```python
from build123d import *


with BuildPart() as part:
    # Sketch2 → Revolve1 (revolve)
    with BuildSketch(Plane.XY, mode=Mode.PRIVATE) as revolve1_sk:
        with BuildLine():
            Line((0, 0), (0, 2.175))
            ThreePointArc((0, 2.175), (-0.292893219, 2.882106781), (-1, 3.175))
            Line((-1, 3.175), (-1.3716, 3.175))
            Line((-1.3716, 3.175), (-1.3716, 1.63195))
            Line((-1.3716, 1.63195), (-7.7216, 1.63195))
            Line((-7.7216, 1.63195), (-7.7216, 2.43195))
            ThreePointArc((-7.7216, 2.43195), (-7.838757288, 2.714792712), (-8.1216, 2.83195))
            Line((-8.1216, 2.83195), (-8.3216, 2.83195))
            ThreePointArc((-8.3216, 2.83195), (-8.604442712, 2.714792712), (-8.7216, 2.43195))
            Line((-8.7216, 2.43195), (-8.7216, 2.38195))
            ThreePointArc((-8.7216, 2.38195), (-8.941269914, 1.851619914), (-9.4716, 1.63195))
            Line((-9.4716, 1.63195), (-9.764947502, 1.63195))
            ThreePointArc((-9.764947502, 1.63195), (-9.895473695, 1.623394861), (-10.023766548, 1.597875826))
            Line((-10.023766548, 1.597875826), (-10.526009523, 1.463300227))
            ThreePointArc((-10.526009523, 1.463300227), (-10.79327667, 1.284718028), (-10.8966, 0.980337314))
            Line((-10.8966, 0.980337314), (-10.8966, 0))
            Line((-10.8966, 0), (0, 0))
        make_face()
    revolve(revolve1_sk.sketch.rotate(Axis((-42.300017882, 0, 0), (1, 0, 0)), 90), axis=Axis((-42.300017882, 0, 0), (1, 0, 0)))


solid = part.part
```
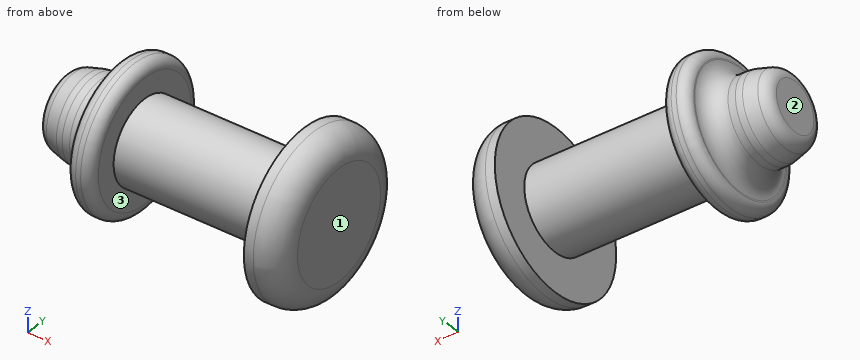
Here's how the part is built. I have some questions about the finished solid (model axes, mm). Face numbers are marked on the shaded views. Coordinates: 2 decimals unless noted, no trailing zeros. Write each loop counter-clockwise with the first axis right and the second up, starting at its lowest first coordinate (ties: lowest second). Pieces come first, ordered by that corner, then holes. Notation, with made-up numbers: M 89.5,-26.5 L 101.5,-26.5 A21 ccw 101.5,-13.5 Z; hole C -38,53.25 d11. An arc over 180 degrees is marked long. Answer as CSV lines item,"result". Start each with the question number.
Q1. Suppose I cut it at B-B, the plane x = -0.5. List the corners of the cut face in (y, z) for me.
Q2. I need wall thicknesses on probe 1 along X at (y, z) = (-1.5, -1.25); probe 2 along X at (y, z) = (-1, -0.25); probe 3 along X at (y, z) = (2, 1.5). Which ranges of each line are inside material? Lowest first, please. Write a range as [from, to].
Q3. Will these pins go through, and if not, where does the flat tip stop? pin 1 Ø1.5 at (x, z) = (-1.5, -1) entering from -Y; pin 2 Ø2 at (x, z) = (-5, -1) entering from +Y; pin 3 Ø2 at (x, y) = (-2.5, 2) entering from +Z; pin 4 Ø1.5 at (x, z) = (-4.5, -2.5) entering from -Y.
Q4. Suppose I cut it at A-A, the plane x = -7.25. List the corners of the cut face in (y, z) for me, then the cut area to 3 significant figures.
Q5. If we mould it in two halves opening along X, with no side actions, what happens to the marked faces 1, 2 and 3? For each: pulls with the +X half, pulls with the -X half, needs draft (parallel to the pull), parting line crosses it, or undercut.
Entries:
1,outline,"C 0,0 d6.08"
2,probe 1,"x = [-8.86, -7.72], [-1.37, 0]"
2,probe 2,"x = [-10.89, 0]"
2,probe 3,"x = [-8.72, -7.73], [-1.37, -0.05]"
3,pin 1,"stops at y = -3.16"
3,pin 2,"stops at y = 1.63"
3,pin 3,"stops at z = 1.29"
3,pin 4,"passes through"
4,outline,"C 0,0 d3.26"
4,area,"8.37 mm²"
5,face 1,"pulls with the +X half"
5,face 2,"pulls with the -X half"
5,face 3,"undercut"
